Build history of the part. All positions in model axes, mm. A direction names the side the tool comes from. Round coordinates to 2 decimals unless told otherwise and drop trailing zeros. Loops run counter-clockwise (first coordinate to the right, second up) from the corner with the lowest first, then second, coordinate; pieces in that order, holes last. Notation, with made-up numbers: (45.25, 70) -> (51.25, 70) arc R20 ccw to (51.25, 86) -> close; hole circle Ø2 at (-26.5, -9.5). An arc over 180 degrees is marked (long way). Put each result on its own line as item: value. Start each with the question number.
```python
from build123d import *

# Parameters (mm, degrees)
PAD065_DEPTH    = 4
PAD066_DEPTH    = 4
PAD067_DEPTH    = 4
SKETCH128_R     = 3.114724
PAD068_DEPTH    = 62
SKETCH129_R     = 2.15
POCKET018_DEPTH = 4.001


with BuildPart() as part:
    # Sketch125 → Pad065 (new body)
    with BuildSketch(Plane.XY):
        Polygon((70, 160), (-70, 160), (-30, 0), (30, 0), align=None)
    extrude(amount=PAD065_DEPTH)

    # Sketch126 (on Face6 of Pad065) → Pad066 (join)
    with BuildSketch(Plane.XY.offset(4)):
        Polygon((-30, 0), (-70, 160), (70, 160), (30, 0), align=None)
        Polygon((-62.315342, 154), (-25.315342, 6), (25.315342, 6), (62.315342, 154), align=None, mode=Mode.SUBTRACT)
    extrude(amount=PAD066_DEPTH)

    # Sketch127 → Pad067 (join)
    with BuildSketch(Plane.YZ.offset(35)):
        Polygon((0, 0), (-3.313708, 0), (-56.346717, 53.033009), (-50.689863, 58.689863), (0, 8), (21, 8), (21, 0), align=None)
    pad067 = extrude(amount=-PAD067_DEPTH)

    # Mirrored006: Pad067 across YZ
    add(pad067.mirror(Plane.YZ))

    # Sketch128 (on Face28 of MultiTransform005) → Pad068 (join)
    with BuildSketch(Plane(origin=(31, 0, 0), x_dir=(0, -1, 0), z_dir=(-1, 0, 0))):
        with Locations((50.926114, 53.082153)):
            Circle(SKETCH128_R)
    extrude(amount=PAD068_DEPTH)

    # Sketch129 (on Face40 of Pad068) → Pocket018 (cut, through all)
    with BuildSketch(Plane.XY.offset(4)):
        with Locations((-6, 14)):
            Circle(SKETCH129_R)
        with Locations((6, 14)):
            Circle(SKETCH129_R)
    extrude(amount=-POCKET018_DEPTH, mode=Mode.SUBTRACT)


with BuildPart() as part_1:
    # Body029 placement: moved
    add(part.part.moved(Location((0, 19.5, -185.5))))


solid = part_1.part
```
Item 1: Wall check: line 1 (Y direction, x = -8, z = -178); line 2 (X direction, y = 33, z = -184); line 3 (Z direction, x = 55, y = 165.5). Give the ranges that are in metal, low to high. Write a range as from..to.
Item 2: Drop flat-ended pins along their axis: pin 1 (4 mm diameter, centred on x = 9, z = -183, fed in from -Y); pin 2 (1 mm diameter, centred on x = -40, y = 148, fed in from +Z). Give the stop position or say it passes through.
Item 3: Cut at B-B on y = 33.5. Write the cut outline in (x, z).
Item 4: Cut at C-C on x = 6. Write the cut outline in (y, z), then the cut area to 3 significant figures.
Item 5: Pull direction X, two halves, no side cores. Call faces 1 (the face through (-35, 1.5, -160.4)), 2 (the face through (-31, -4, -158)), 3 (the face through (30.5, 21.5, -181.6)), 4 (the face through (33, -6, -152)): +X half, -X half, draft (parallel to the pull), parting line (faces both ways), or undercut.
Item 6: Cut at A-A on z = -171. Write the cut outline in (x, y).
Item 7: Cut at D-D on y = 134.5. Write the cut outline in (x, z), then the cut area to 3 significant figures.
Item 8: 3-axis set-ups, long thin cutter, end or side, ignore diameter. For faces 5 (the face through (43.556, 98.464, -179.528)), 6 (the face through (-33.028, -9.959, -159.355)), 7 (the face through (0, 19.5, -182)): which of +Z, -Z, +X, -X, +Y, -Y reach the whole face in a straight line?
Ans:
1. line 1: y = 19.5..25.5, 173.5..179.5
1. line 2: x = -35..-8.09, -3.91..3.91, 8.09..35
1. line 3: z = -185.5..-181.5
2. pin 1: stops at y = 19.5
2. pin 2: stops at z = -181.5
3. outline: (-35, -185.5) -> (-8.15, -185.5) -> (-8.15, -181.5) -> (-27.32, -181.5) -> (-27.32, -177.5) -> (-35, -177.5) -> close; (-3.85, -185.5) -> (3.85, -185.5) -> (3.85, -181.5) -> (-3.85, -181.5) -> close; (8.15, -185.5) -> (35, -185.5) -> (35, -177.5) -> (27.32, -177.5) -> (27.32, -181.5) -> (8.15, -181.5) -> close
4. outline: circle Ø6.23 at (-31.43, -132.42); (19.5, -185.5) -> (31.35, -185.5) -> (31.35, -181.5) -> (25.5, -181.5) -> (25.5, -177.5) -> (19.5, -177.5) -> close; (35.65, -185.5) -> (179.5, -185.5) -> (179.5, -177.5) -> (173.5, -177.5) -> (173.5, -181.5) -> (35.65, -181.5) -> close
4. area: 701 mm2
5. face 1: -X half
5. face 2: undercut
5. face 3: undercut
5. face 4: draft
6. outline: (-35, 1.69) -> (-31, 1.69) -> (-31, 13) -> (-35, 13) -> close; (31, 1.69) -> (35, 1.69) -> (35, 13) -> (31, 13) -> close
7. outline: (-58.75, -185.5) -> (58.75, -185.5) -> (58.75, -177.5) -> (52.57, -177.5) -> (52.57, -181.5) -> (-52.57, -181.5) -> (-52.57, -177.5) -> (-58.75, -177.5) -> close
7. area: 519 mm2
8. face 5: +Z
8. face 6: -Z, +X, -X, -Y
8. face 7: +Z, -Z, -Y
